Check sheet for the drawn part. Datum: minimum x, y, z corner. Units: mm. A direction names the side the tool comes from. Round coordinates to 2 decimals unless told otherwise and drop trailing zeros. Loops run counter-clockwise (first coordinate to the right, second up) from the corner with the lowest first, then second, coordinate; pieces in that order, holes last. Notation, with made-up numbers: (25, 21) -> (55, 21) arc R23 ccw to (55, 29) -> close; hole circle Ø11 at (-12, 26.25). An arc over 180 degrees is marked (long way). Return JSON: item names as keys, results as strings.
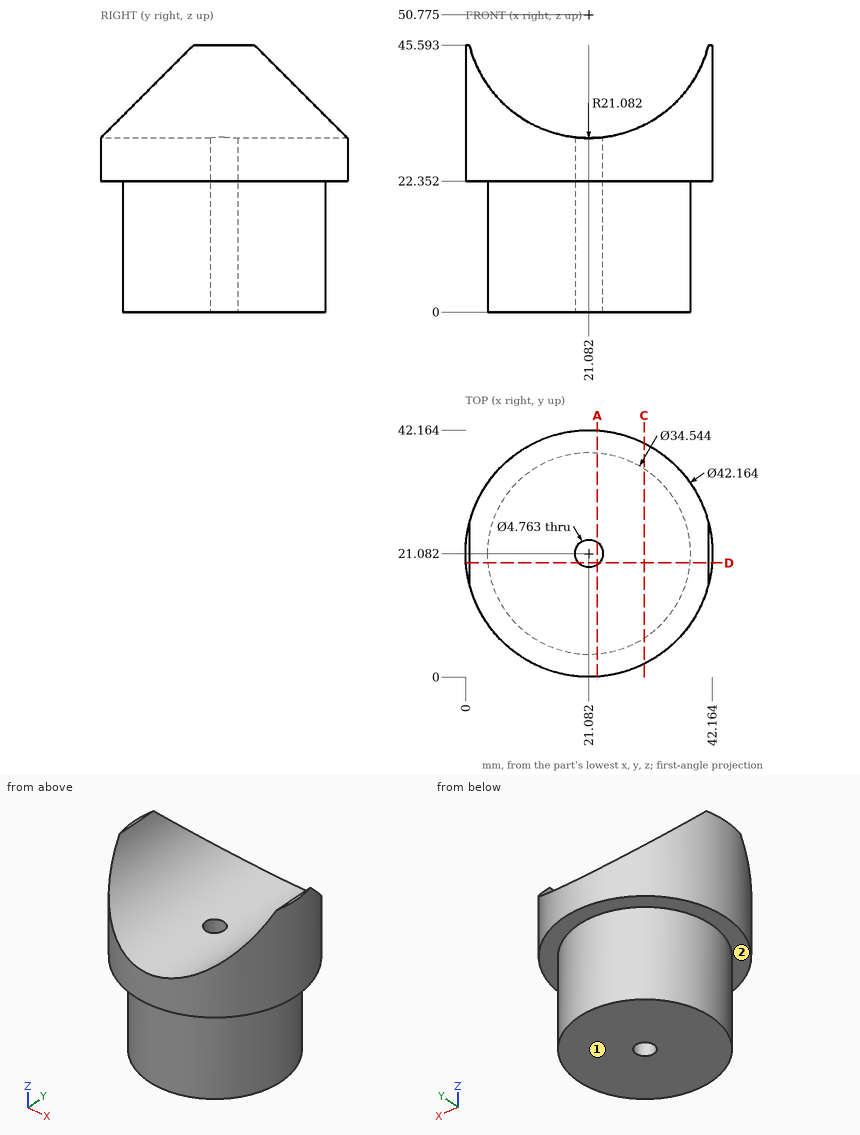
Q1. Section check A-A (x = 22.5). Record the boundary of the cut face in (y, z) (1 decimal).
Results list:
{"outline": "(0, 22.4) -> (3.9, 22.4) -> (3.9, 0) -> (19.2, 0) -> (19.2, 29.7) -> (0, 29.7) -> close; (23, 0) -> (38.3, 0) -> (38.3, 22.4) -> (42.1, 22.4) -> (42.1, 29.7) -> (23, 29.7) -> close"}
Q2. Section check D-D (y = 19.5). Record the boundary of the cut face in (x, z) (1 decimal), then the cut area to 3 significant figures.
Results list:
{"outline": "(0.1, 22.4) -> (3.9, 22.4) -> (3.9, 0) -> (19.3, 0) -> (19.3, 29.8) arc R21.1 cw to (0.6, 45.6) -> (0.1, 45.6) -> close; (22.9, 0) -> (38.3, 0) -> (38.3, 22.4) -> (42.1, 22.4) -> (42.1, 45.6) -> (41.5, 45.6) arc R21.1 cw to (22.9, 29.8) -> close", "area": "1,160 mm^2"}
Q3. Section check C-C (x = 30.5). Record the boundary of the cut face in (y, z).
Results list:
{"outline": "(2.22, 22.35) -> (6.6, 22.35) -> (6.6, 0) -> (35.56, 0) -> (35.56, 22.35) -> (39.94, 22.35) -> (39.94, 31.91) -> (2.22, 31.91) -> close"}
Q4. Go/stop test with flat-tipped pins: pin 1 (5 mm diameter, centred on x = 37, z = 21.5, fed in from +Y); pin 2 (6 mm diameter, centred on x = 17.5, y = 25.5, fed in from +Z); pin 3 (8 mm diameter, centred on x = 24.5, z = 18, fed in from -Y). Record where each tip stops, or that it passes through.
Results list:
{"pin 1": "y = 37.22", "pin 2": "z = 30.75", "pin 3": "y = 3.81"}
Q5. Material ranges on line 1 (X direction, y = 25.5, z = 37.5) (1 decimal); line 2 (X direction, y = 29, z = 37) (1 decimal); line 3 (Z direction, x = 36.5, y = 22) (1 decimal), recorded low to high.
Results list:
{"line 1": "0.5 to 4.7, 37.5 to 41.7", "line 2": "1.5 to 5.1, 37 to 40.6", "line 3": "0 to 36.4"}
Q6. Tool access check on the marked faces 1 and 2. Record the directions out of +Z, -Z, +X, -X, +Y, -Y that give a thin tool (end or side, any length) a straight path to the whole face; none if there is none.
Results list:
{"face 1": "-Z, +X, -X, +Y, -Y", "face 2": "-Z"}
